from build123d import *

# Parameters (mm, degrees)
SKETCH1_R          = 19
BASE_EXTRUDE_DEPTH = 36
SCALE1_SCALE       = 2.5
SCALE2_SCALE       = 1.2


with BuildPart() as part:
    # Sketch1 → Base-Extrude (new body)
    with BuildSketch(Plane.XY):
        Circle(SKETCH1_R)
    extrude(amount=BASE_EXTRUDE_DEPTH)


with BuildPart() as part_1:
    # Scale1: scaled about (0, 0, 18)
    add(part.part.scale(SCALE1_SCALE).moved(Location((0, 0, -27))))


with BuildPart() as part_2:
    # Scale2: scaled about (0, 0, 18)
    add(part_1.part.scale(SCALE2_SCALE).moved(Location((0, 0, -3.6))))


solid = part_2.part
Design review of the part built by this model. Coordinates are the model's own, in mm. Round coordinates to 2 decimals unless told otherwise and drop trailing zeros. Loops run counter-clockwise (first coordinate to the right, second up) from the corner with the lowest first, then second, coordinate; pieces in that order, holes last. Notation, with made-up numbers: (-22.75, -19.75) - (1.25, -19.75) arc R19 cw to (1.25, -12.75) - close; hole circle Ø2 at (12, -26). An arc over 180 degrees is marked (long way). One line per question, with ' | ' between items.
1. We need section A-A, the plane z = -19.5. State the section outline as (x, y) points, and give its area (3 significant figures).
Results are:
outline: circle Ø114 at (0, 0) | area: 10,200 mm²
2. For L1, parallel to Y at x = 0, z = 67; L2, parallel to X at y = -6.5, z = 26; L3, parallel to X at y = -20, z = 13.5, list the stretches that pass through material, from the lowest coordinate up. Write a range as [from, to].
Results are:
L1: y = [-57, 57] | L2: x = [-56.63, 56.63] | L3: x = [-53.38, 53.38]
3. Draft analysis for pull direction X (two halves, no side actions). For faces 1 (the face through (-1, 1, 72)), 2 (the face through (52.654, -21.831, 17.244)), state which applies: released by +X, released by -X, zero draft, split by the parting line, or undercut.
Results are:
face 1: zero draft | face 2: split by the parting line
4. We need section C-C, the plane y = 16. State the section outline as (x, z) points.
Results are:
outline: (-54.71, -36) - (54.71, -36) - (54.71, 72) - (-54.71, 72) - close
5. Clearance check with flat-ended pins moving along their axes: P1, Ø12, axis at x = -18, z = 48.5, coming from the +Y side; P2, Ø12, axis at y = 45.5, z = -10.5, coming from the -X side; P3, Ø5, axis at y = -14, z = -9, coming from the -X side. State where each tip first meets the part, or that it passes through.
Results are:
P1: stops at y = 55.72 | P2: stops at x = -41.09 | P3: stops at x = -55.83
6. We need section B-B, the plane x = -18. State the section outline as (y, z) points.
Results are:
outline: (-54.08, -36) - (54.08, -36) - (54.08, 72) - (-54.08, 72) - close
